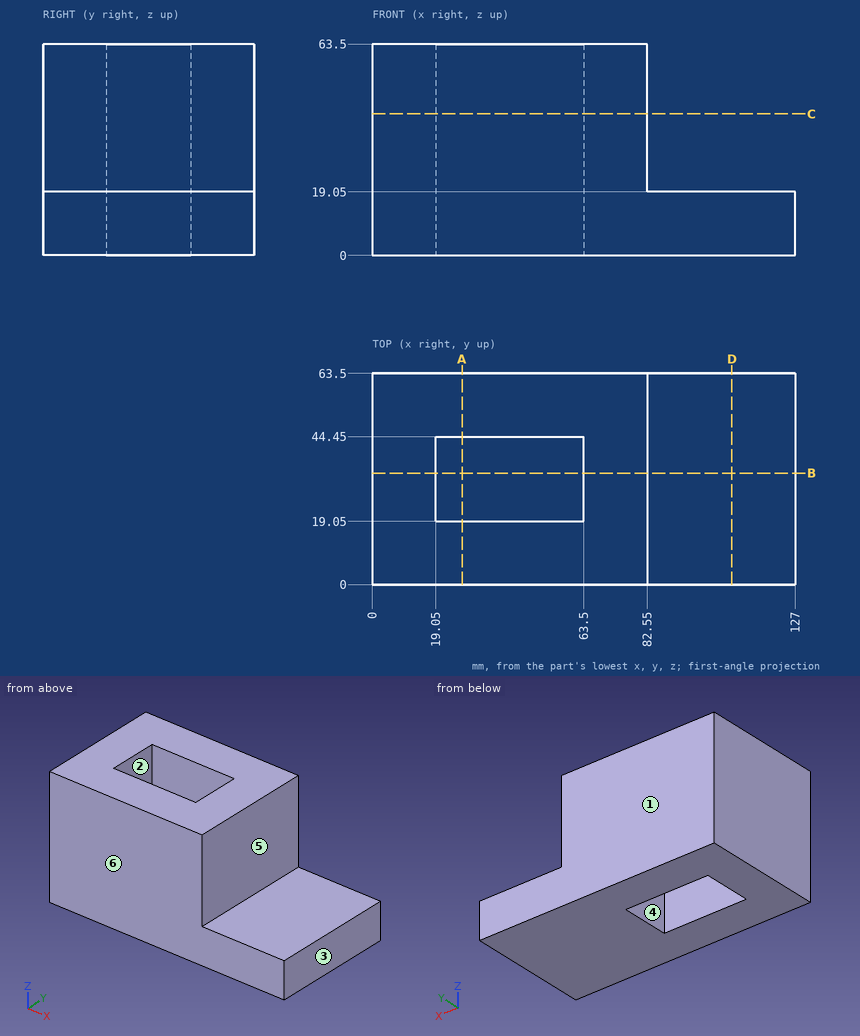
Can you work these out from the drawing? Everything is in mm from the part's minimum corner. A direction names the side the tool comes from. Give positions to 0.01 mm unless a question says otherwise; leave off trailing zeros. Order: outer loops, then holes, each group sorted by start corner. A loop starts at its lowest first (then second) coordinate and runs counter-clockwise, first axis right, second up. Notation, with made-up numbers: M 42.25,-21 L 100.25,-21 A36 ccw 100.25,15 Z; hole C 39,23.25 d10. An arc over 180 degrees is marked long. Use a Markdown table: item, result. Add a question column.
1. I need wall thicknesses on probe 1 along X at (y, z) = (39, 31.5); probe 2 along Y at (x, z) = (27.5, 7); probe 3 along Z at (x, y) = (122.5, 50). Which ranges of each line are inside material? Lowest first, please. Write a range as from..to.
2. Suppose I cut it at D-D (x = 108). List the corners of the cut face in (y, z) for me.
3. For pin 1 Ø1 at (y, z) = (40.5, 44.5) entering from +X; pin 2 Ø1 at (x, y) = (88, 29) entering from +Z; pin 3 Ø8 at (x, z) = (87, 40) entering from -Y, each with a flat end and sliding along its axis, tell me the tip position at first contact or that it passes through.
4. If we mould it in two halves opening along Y, with no side actions, what happens to the marked faces 1, 2 and 3? For each: +Y half, -Y half, draft (parallel to the pull), parting line (faces both ways), or undercut.
5. Suppose I cut it at C-C (z = 42.5). List the corners of the cut face in (x, y) for me, and give its area (3 significant figures).
6. Suppose I cut it at B-B (y = 33.5). List the corners of the cut face in (x, z) for me, and give its area (3 significant figures).
7. Suppose I cut it at A-A (x = 27). List the corners of the cut face in (y, z) for me, and give its area (3 significant figures).
8. On a 3-axis mill with a long thin cutter (end or side, diameter ignored), from which of +Z, -Z, +X, -X, +Y, -Y can I reach the whole of each face in a straight line? I mean the marked faces 4, 5 and 6. Say none if no direction works.
Results list:
| question | item | result |
|---|---|---|
| 1 | probe 1 | x = 0..19.05, 63.5..82.55 |
| 1 | probe 2 | y = 0..19.05, 44.45..63.5 |
| 1 | probe 3 | z = 0..19.05 |
| 2 | outline | M 0,0 L 63.5,0 L 63.5,19.05 L 0,19.05 Z |
| 3 | pin 1 | stops at x = 82.55 |
| 3 | pin 2 | stops at z = 19.05 |
| 3 | pin 3 | passes through |
| 4 | face 1 | +Y half |
| 4 | face 2 | undercut |
| 4 | face 3 | draft |
| 5 | outline | M 0,0 L 82.55,0 L 82.55,63.5 L 0,63.5 Z; hole M 19.05,19.05 L 63.5,19.05 L 63.5,44.45 L 19.05,44.45 Z |
| 5 | area | 4,110 mm² |
| 6 | outline | M 0,0 L 19.05,0 L 19.05,63.5 L 0,63.5 Z; M 63.5,0 L 127,0 L 127,19.05 L 82.55,19.05 L 82.55,63.5 L 63.5,63.5 Z |
| 6 | area | 3,270 mm² |
| 7 | outline | M 0,0 L 19.05,0 L 19.05,63.5 L 0,63.5 Z; M 44.45,0 L 63.5,0 L 63.5,63.5 L 44.45,63.5 Z |
| 7 | area | 2,420 mm² |
| 8 | face 4 | +Z, -Z |
| 8 | face 5 | +Z, +X, +Y, -Y |
| 8 | face 6 | +Z, -Z, +X, -X, -Y |
